Geometry check sheet. Reference: the model listing, model coordinates, mm. Face numbers are marked on the shaded views. A direction names the side the tool comes from. Round coordinates to 2 decimals unless told otherwise and drop trailing zeros. Write each loop counter-clockwise with the first axis right and the second up, starting at its lowest first coordinate (ties: lowest second). Pieces come first, ordered by that corner, then holes. Notation, with made-up numbers: M -11,30 L 48,30 A11 cw 48,49 Z; hole C -13,-1.5 d10. An arc over 180 degrees is marked long. Use a Markdown table: item, result.
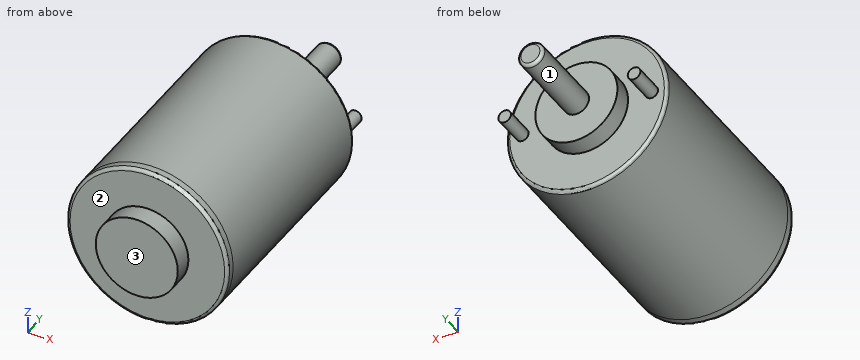
```python
from build123d import *

# Parameters (mm, degrees)
SKETCH2_R            = 25.5
BOSS_EXTRUDE1_DEPTH  = 32.5
SKETCH3_R            = 25.5
BOSS_EXTRUDE2_DEPTH  = 3
FILLET1_R            = 1
SKETCH4_R            = 13
BOSS_EXTRUDE3_DEPTH  = 6
FILLET1_OF_MIRROR1_R = 1
SKETCH5_R            = 4
BOSS_EXTRUDE4_DEPTH  = 26
SKETCH6_R            = 2
BOSS_EXTRUDE5_DEPTH  = 10
FILLET2_R            = 1


with BuildPart() as part:
    # Sketch2 → Boss-Extrude1 (new body, symmetric)
    with BuildSketch(Plane(origin=(0, 0, 0), x_dir=(1, 0, 0), z_dir=(0, 1, 0))):
        Circle(SKETCH2_R)
    extrude(amount=BOSS_EXTRUDE1_DEPTH, both=True)

    # Sketch3 → Boss-Extrude2 (add)
    with BuildSketch(Plane(origin=(0, 32.5, 0), x_dir=(1, 0, 0), z_dir=(0, 1, 0))):
        Circle(SKETCH3_R)
    boss_extrude2 = extrude(amount=BOSS_EXTRUDE2_DEPTH)

    # Fillet1
    fillet1_edges = [part.edges().sort_by_distance(p)[0] for p in [
        (-25.5, 35.5, 0),
    ]]
    fillet(fillet1_edges, radius=FILLET1_R)

    # Sketch4 → Boss-Extrude3 (add)
    with BuildSketch(Plane(origin=(0, 35.5, 0), x_dir=(1, 0, 0), z_dir=(0, 1, 0))):
        Circle(SKETCH4_R)
    boss_extrude3 = extrude(amount=BOSS_EXTRUDE3_DEPTH)

    # Mirror1: Boss-Extrude2, Boss-Extrude3 across plane
    add(boss_extrude2.mirror(Plane.ZX))
    add(boss_extrude3.mirror(Plane.ZX))

    # Fillet1 of Mirror1
    fillet1_of_mirror1_edges = [part.edges().sort_by_distance(p)[0] for p in [
        (-25.5, -35.5, 0),
    ]]
    fillet(fillet1_of_mirror1_edges, radius=FILLET1_OF_MIRROR1_R)

    # Sketch5 → Boss-Extrude4 (add)
    with BuildSketch(Plane(origin=(0, 41.5, 0), x_dir=(1, 0, 0), z_dir=(0, 1, 0))):
        Circle(SKETCH5_R)
    extrude(amount=BOSS_EXTRUDE4_DEPTH)

    # Sketch6 → Boss-Extrude5 (add)
    with BuildSketch(Plane(origin=(0, 35.5, 0), x_dir=(1, 0, 0), z_dir=(0, 1, 0))):
        with Locations((-20.5, 0)):
            Circle(SKETCH6_R)
        with Locations((20.5, 0)):
            Circle(SKETCH6_R)
    extrude(amount=BOSS_EXTRUDE5_DEPTH)

    # Fillet2
    fillet2_edges = [part.edges().sort_by_distance(p)[0] for p in [
        (-4, 67.5, 0),
    ]]
    fillet(fillet2_edges, radius=FILLET2_R)


solid = part.part
```
Item 1: Cross-section at A-A, the plane x = 0. Record the cut outline in (y, z), and give its area (3 significant figures).
Outcome:
| item | result |
|---|---|
| outline | M -41.5,-13 L -35.5,-13 L -35.5,-24.5 A1 ccw -34.5,-25.5 L 34.5,-25.5 A1 ccw 35.5,-24.5 L 35.5,-13 L 41.5,-13 L 41.5,-4 L 66.5,-4 A1 ccw 67.5,-3 L 67.5,3 A1 ccw 66.5,4 L 41.5,4 L 41.5,13 L 35.5,13 L 35.5,24.5 A1 ccw 34.5,25.5 L -34.5,25.5 A1 ccw -35.5,24.5 L -35.5,13 L -41.5,13 Z |
| area | 4,140 mm2 |
Item 2: Go/stop test with flat-tipped pins: pin 1 (1 mm diameter, centred on y = 40, z = -1.5, fed in from -X); pin 2 (10 mm diameter, centred on x = -16.5, z = 15.5, fed in from -Y); pin 3 (1.5 mm diameter, centred on x = 10.5, y = 16.5, fed in from +Z). Record where each tip stops, or that it passes through.
Outcome:
| item | result |
|---|---|
| pin 1 | stops at x = -22.23 |
| pin 2 | stops at y = -35.5 |
| pin 3 | stops at z = 23.56 |
Item 3: Access from +Z, -Z, +X, -X, +Y, -Y to the whole of each face (thin tool, end or side, straight path). Record for the marked faces 1, 2 and 3.
Outcome:
| item | result |
|---|---|
| face 1 | +Y |
| face 2 | -Y |
| face 3 | +Z, -Z, +X, -X, -Y |
Item 4: Cross-section at D-D, the plane y = 60. Record the cut outline in (x, z).
Outcome:
| item | result |
|---|---|
| outline | C 0,0 d8 |
Item 5: Cross-section at C-C, the plane y = 38. Record the cut outline in (x, z), and give its area (3 significant figures).
Outcome:
| item | result |
|---|---|
| outline | C -20.5,0 d4; C 0,0 d26; C 20.5,0 d4 |
| area | 556 mm2 |
Item 6: Material ranges on line 1 along Y through (x, z) = (-5, 11.5); line 2 along Z through (x, y) = (-1, 8); line 3 along Y through (x, z) = (19, 10.5), recorded low to high. Write a range as from..to.
Outcome:
| item | result |
|---|---|
| line 1 | y = -41.5..41.5 |
| line 2 | z = -25.48..25.48 |
| line 3 | y = -35.5..35.5 |
